Geometry check sheet. Reference: the model listing, model coordinates, mm. A direction names the side the tool comes from. Round coordinates to 2 decimals unless told otherwise and drop trailing zeros. Write each loop counter-clockwise with the first axis right and the second up, starting at its lowest first coordinate (ties: lowest second). Pieces come first, ordered by that corner, then holes.
Item 1: Access from +Z, -Z, +X, -X, +Y, -Y to the whole of each face (thin tool, end or side, straight path). Record for faces 4 (the face through (-0.124, -20.268, 55.443)), 5 (the face through (17.153, 5.402, 36.35)).
Item 2: Cross-section at D-D (z = 8). Enter the section's corners in (x, y).
Item 3: Depth check by flat-ended pin: P1, Ø12, axis at x = 14, y = 11, coming from the +Z side; P2, Ø1, axis at x = -8.5, y = 10, coming from the +Z side; P3, Ø1.5, axis at x = -2, z = 44, coming from the +Y side; P4, Ø10, axis at y = 16.5, z = 21.5, coming from the +X side. Enter the tip coordinate at first touch or a pass-through.
Item 4: Cross-section at C-C (x = 16). Enter the section's corners in (y, z), then the cut area to 3 significant figures.
Item 5: Draft check along Y on faces 1 (the face through (0, 0, 11)), 2 (the face through (18.5, 0.1, 61)), 3 (the face through (-5.073, -22.845, 30.073)). Enter one of: pulls with the +Y half, pulls with the -Y half, needs draft (parallel to the pull), parting line crosses it, or undercut.
Item 6: Cross-section at B-B (y = 0). Enter the section's corners in (x, z), then the cut area to 3 significant figures.
Item 7: Cross-section at A-A (z = 26). Enter the section's corners in (x, y).
Item 8: Scan lines: probe 1 along X at (y, z) = (0, 45); probe 2 along Z at (x, y) = (-6.5, 3). Record each from-to range of solid material in increasing order.
from build123d import *

# Parameters (mm, degrees)
F0_R     = 23.401279
F1_DEPTH = 61
F3_R     = 17.983402
F4_DEPTH = 50
F6_R     = 5.743652
F7_DEPTH = 63.5


with BuildPart() as f1:
    # F0 (on Top) → F1 (new body)
    with BuildSketch(Plane.XY):
        Circle(F0_R)
    extrude(amount=F1_DEPTH)

    # F3 (on offset) → F4 (cut)
    with BuildSketch(Plane.XY.offset(61)):
        Circle(F3_R)
    extrude(amount=-F4_DEPTH, mode=Mode.SUBTRACT)

    # F6 (on offset) → F7 (cut)
    with BuildSketch(Plane.XZ.offset(25)):
        with Locations((0, 61.185386)):
            Circle(F6_R)
    extrude(amount=-F7_DEPTH, mode=Mode.SUBTRACT)


solid = f1.part
Resolved:
1. face 4: +Z, +Y, -Y
1. face 5: +Z
2. outline: circle Ø46.8 at (0, 0)
3. P1: stops at z = 61
3. P2: stops at z = 11
3. P3: stops at y = 23.37
3. P4: stops at x = 20.38
4. outline: (-17.08, 0) - (17.08, 0) - (17.08, 61) - (8.21, 61) - (8.21, 11) - (-8.21, 11) - (-8.21, 61) - (-17.08, 61) - close
4. area: 1,260 mm2
5. face 1: undercut
5. face 2: needs draft
5. face 3: parting line crosses it
6. outline: (-23.4, 0) - (23.4, 0) - (23.4, 61) - (17.98, 61) - (17.98, 11) - (-17.98, 11) - (-17.98, 61) - (-23.4, 61) - close
6. area: 1,060 mm2
7. outline: circle Ø46.8 at (0, 0); hole circle Ø35.97 at (0, 0)
8. probe 1: x = -23.4 to -17.98, 17.98 to 23.4
8. probe 2: z = 0 to 11
